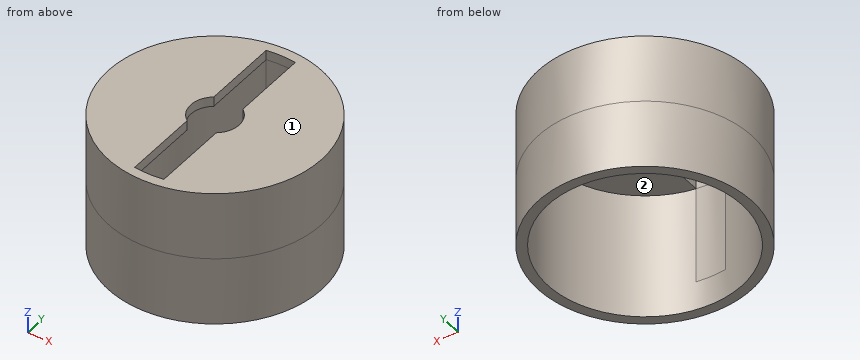
Autodesk Inventor part; units mm, degrees
ref_plane "YZ Plane" through (0, 0, 0) normal (1, 0, 0) x (0, 1, 0)
ref_plane "XZ Plane" through (0, 0, 0) normal (0, 1, 0) x (-1, 0, 0)
ref_plane "XY Plane" through (0, 0, 0) normal (0, 0, 1) x (1, 0, 0)
sketch "Skizze1" plane through (0, 0, 0) normal (0, 0, 1) x (1, 0, 0)
  circle A0 centre (0, 0) radius 11
  dimension "d0" = 22
extrude "Extrusion1" add sketch "Skizze1" along normal mid plane 14
sketch "Skizze2" plane through (0, 0, -7) normal (0, 0, -1) x (-1, 0, 0)
  circle A0 centre (0, 0) radius 10
  circle A1 centre (0, 0) radius 11
  dimension "d3" = 1
extrude "Extrusion2" cut sketch "Skizze2" against normal blind 13 contours A0
sketch "Skizze3" plane through (0, 0, 7) normal (0, 0, 1) x (1, 0, 0)
  circle A0 centre (0, 0) radius 2.5
  circle A1 centre (0, 0) radius 10
  line L0 (1.5, -9.8869) -> (1.5, 9.8869)
  line L1 (-1.5, -9.8869) -> (-1.5, 9.8869)
  point P0 (-1.5, 2)
  point P1 (-1.5, -2)
  point P2 (1.5, -2)
  point P3 (1.5, 2)
  dimension "d6" = 5
  dimension "d7" = 3
  dimension "d8" = 1.5
extrude "Extrusion3" cut sketch "Skizze3" against normal blind 11 contours A0 L0 | L0 A0 L1 | A0 L1 A1 L0 | L0 A1 L1 A0 | L1 A0
properties part number "LED-Schirm"
Geometry check sheet. Reference: the model listing, model coordinates, mm. Face numbers are marked on the shaded views. Coordinates: 2 decimals unless noted, no trailing zeros. Loops run counter-clockwise (first coordinate to the right, second up) from the corner with the lowest first, then second, coordinate; pieces in that order, holes last. Notation, with made-up numbers: (-21.75, 86.5) - (17.25, 86.5) arc R27 cw to (17.25, 125.5) - close; hole circle Ø2 at (8.5, 57.25). An arc over 180 degrees is marked (long way). Use one line per item in the form item = value. Start each with the question number.
Item 1: Mould release check, pull along Y, two halves, no side actions. Record for the marked faces 1 and 2: +Y half, -Y half, draft (parallel to the pull), parting line (faces both ways), or undercut.
Item 2: Section check A-A, the plane x = 0. Enter the section's corners in (y, z), and give its area (3 significant figures).
Item 3: Section check C-C, the plane z = 2.25. Enter the section's corners in (x, y).
Item 4: Section check B-B, the plane y = 0. Enter the section's corners in (x, z), and give its area (3 significant figures).
Item 5: Gauge pin test, flat ends, axial feed: pin 1 (0.5 mm diameter, centred on y = 5, z = 6.5, fed in from -X); pin 2 (4 mm diameter, centred on y = -1.5, z = -1, fed in from -X); pin 3 (0.5 mm diameter, centred on y = 4, z = 6.5, fed in from +X); pin 4 (6 mm diameter, centred on x = 1, y = 1, fed in from -Z). Record the tip position at first contact, or that the pin passes through.
Item 6: Thickness scan on probe 1 along Y at (x, z) = (0, -1); probe 2 along Y at (x, z) = (7.5, 4.5); probe 3 along Z at (x, y) = (2, -7). Record the ranges inside material, lowest first.
Item 7: Section check D-D, the plane x = -8.5. Enter the section's corners in (y, z), and give its area (3 significant figures).
Computed:
q1.face_1 = draft
q1.face_2 = undercut
q2.outline = (-11, -7) - (-10, -7) - (-10, 7) - (-11, 7) - close; (10, -7) - (11, -7) - (11, 7) - (10, 7) - close
q2.area = 28.0 mm2
q3.outline = circle Ø22 at (0, 0); hole circle Ø20 at (0, 0)
q4.outline = (-11, -7) - (-10, -7) - (-10, 6) - (-2.5, 6) - (-2.5, 7) - (-11, 7) - close; (2.5, 6) - (10, 6) - (10, -7) - (11, -7) - (11, 7) - (2.5, 7) - close
q4.area = 43.0 mm2
q5.pin_1 = -9.92
q5.pin_2 = -11
q5.pin_3 = 10.34
q5.pin_4 = 6
q6.probe_1 = -11 to -10, 10 to 11
q6.probe_2 = -8.05 to -6.61, 6.61 to 8.05
q6.probe_3 = 6 to 7
q7.outline = (-6.98, -7) - (-5.27, -7) - (-5.27, 6) - (5.27, 6) - (5.27, -7) - (6.98, -7) - (6.98, 7) - (-6.98, 7) - close
q7.area = 58.5 mm2
